For this review, take the finished solid that the model builds, in its own axes (mm). A direction names the side the tool comes from. Coordinates: 2 decimals unless noted, no trailing zeros. Loops run counter-clockwise (first coordinate to the right, second up) from the corner with the lowest first, then second, coordinate; pieces in that order, holes last. Notation, with made-up numbers: M 64.25,20 L 114.25,20 A28 cw 114.25,52 Z; hole C 87.5,33.25 d6. An arc over 180 degrees is marked long. Write item = value, one per line.
from build123d import *

# Parameters (mm, degrees)
SKETCH1_W           = 25.5
SKETCH1_H           = 118
BOSS_EXTRUDE1_DEPTH = 4.9
BOSS_EXTRUDE5_DEPTH = 50
SKETCH2_R           = 1.95
CUT_EXTRUDE1_DEPTH  = 10


with BuildPart() as part:
    # Sketch1 → Boss-Extrude1 (new body)
    with BuildSketch(Plane(origin=(0, 0, 0), x_dir=(1, 0, 0), z_dir=(0, 1, 0))):
        Rectangle(SKETCH1_W, SKETCH1_H)
    extrude(amount=BOSS_EXTRUDE1_DEPTH)

    # Sketch5 → Boss-Extrude5 (add)
    with BuildSketch(Plane.XY.offset(59)):
        Polygon((-4.9, 0), (-4.9, -5.2), (-8.8, -5.2), (-4.9, -10), (4.9, -10), (8.8, -5.2), (4.9, -5.2), (4.9, 0), align=None)
    extrude(amount=-BOSS_EXTRUDE5_DEPTH)

    # Sketch2 → Cut-Extrude1 (cut)
    with BuildSketch(Plane(origin=(0, 4.9, 0), x_dir=(1, 0, 0), z_dir=(0, 1, 0))):
        with Locations((1.25, 56)):
            Circle(SKETCH2_R)
        with Locations((1.25, -56)):
            Circle(SKETCH2_R)
    extrude(amount=-CUT_EXTRUDE1_DEPTH, mode=Mode.SUBTRACT)


solid = part.part
Q1. Add section B-B (x = 1.25). Write out the cut boundary in (y, z).
Solved:
outline = M -10,9 L 0,9 L 0,-54.05 L 4.9,-54.05 L 4.9,54.05 L -5.1,54.05 L -5.1,57.95 L 4.9,57.95 L 4.9,59 L -10,59 Z; M 0,-59 L 4.9,-59 L 4.9,-57.95 L 0,-57.95 Z
Q2. Add section C-C (z = 56). Write out the cut boundary in (x, y), and give its area (3 significant figures).
Solved:
outline = M -12.75,0 L -4.9,0 L -4.9,-5.2 L -8.8,-5.2 L -4.9,-10 L 4.9,-10 L 8.8,-5.2 L 4.9,-5.2 L 4.9,0 L 12.75,0 L 12.75,4.9 L 3.2,4.9 L 3.2,-5.1 L -0.7,-5.1 L -0.7,4.9 L -12.75,4.9 Z
area = 203 mm²
Q3. Add section A-A (z = -56). Write out the cut boundary in (x, y), and give its area (3 significant figures).
Solved:
outline = M -12.75,0 L -0.7,0 L -0.7,4.9 L -12.75,4.9 Z; M 3.2,0 L 12.75,0 L 12.75,4.9 L 3.2,4.9 Z
area = 106 mm²
Q4. Draft analysis for pull direction Z (two halves, no side actions). For faces 1 (the face through (4.9, -3, 34)), 2 (the face through (0, -5, 9)), 3 (the face through (0.996, 2.484, -57.933)), state which applies: +Z half, -Z half, draft (parallel to the pull), parting line (faces both ways), or undercut.
Solved:
face_1 = draft
face_2 = -Z half
face_3 = undercut
Q5. For pin 1 Ø8 at (x, y) = (3.5, -5.5) entering from -Z; pin 2 Ø4 at (y, z) = (-2.5, 38) entering from -X; pin 3 Ø7.5 at (x, z) = (4, -1) entering from -Y; pin 4 Ø5.5 at (y, z) = (-2, 30) entering from +X, all flat-tipped, find the tip position at first contact; note any pin that passes through.
Solved:
pin_1 = 9
pin_2 = -4.9
pin_3 = 0
pin_4 = 12.75
Q6. For line 1 along Z through (x, y) = (1.25, 2.25); line 2 along X through (y, z) = (2.65, -56); line 3 along Z through (x, y) = (2.75, 2), list the stretches that pass through material, from the lowest coordinate up.
Solved:
line_1 = -59 to -57.95, -54.05 to 54.05, 57.95 to 59
line_2 = -12.75 to -0.7, 3.2 to 12.75
line_3 = -59 to -57.25, -54.75 to 54.75, 57.25 to 59
Q7. Machinability: for faces 4 (the face through (1, -5.1, 56)), 5 (the face through (0, 0, -1)), 6 (the face through (7, -5.2, 34)), 7 (the face through (-7, -5.2, 34)), which of the approach directions +Z, -Z, +X, -X, +Y, -Y give a long, thin tool a straight path to every point of the face, cutting with its end or side? Answer none if there is none.
Solved:
face_4 = +Y
face_5 = -Z
face_6 = +Z, -Z, +X
face_7 = +Z, -Z, -X
Q8. Add section D-D (y = -2.75). Write out the cut boundary in (x, z), and give its area (3 significant figures).
Solved:
outline = M -4.9,9 L 4.9,9 L 4.9,59 L -4.9,59 Z; hole C 1.25,56 d3.9
area = 478 mm²
